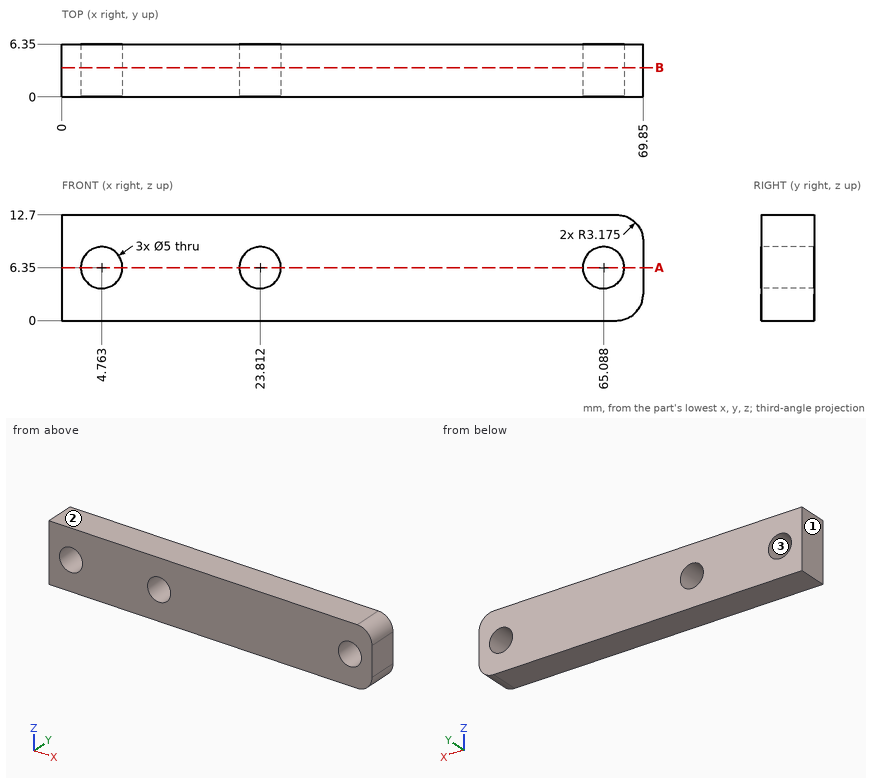
Here's the drawing with two shaded views (mm, measured from the low corner). I have some questions. Coordinates: 2 decimals unless noted, no trailing zeros. Loops run counter-clockwise (first coordinate to the right, second up) from the corner with the lowest first, then second, coordinate; pieces in that order, holes last. Notation, with made-up numbers: (-7.75, -13.5) -> (1.25, -13.5) arc R20 ccw to (1.25, 6.5) -> close; hole circle Ø10 at (-26.5, -14). An arc over 180 degrees is marked (long way). Answer as a JSON object with one key per item and string values.
1) Thinking about a two-plate mould opening in Z: for the marked faces 1, 2 and 3, which applies, pulls with the +Z half, pulls with the -Z half, needs draft (parallel to the pull), parting line crosses it, or undercut?
Results:
{"face 1": "needs draft", "face 2": "pulls with the +Z half", "face 3": "undercut"}
2) If I drill on line 1 (Z direction, x = 24, y = 2.25); line 2 (X direction, y = 2.25, z = 3) (1 decimal); line 3 (X direction, y = 5.5, z = 10.75) (1 decimal), over which ranges is the centre line in solid material (lowest first)?
Results:
{"line 1": "z = 0 to 3.86, 8.84 to 12.7", "line 2": "x = 0 to 69.8", "line 3": "x = 0 to 69.6"}
3) Imagine slicing it at B-B (y = 3.5). Count the separate pieces of the cut face and the enclosed holes in it, then the cut area to 3 significant figures.
Results:
{"separate pieces": "1", "enclosed holes": "3", "area": "824 mm^2"}
4) Imagine slicing it at A-A (z = 6.35). Please give me the cut outline in (x, y), then the cut area to 3 significant figures.
Results:
{"outline": "(0, 0) -> (2.26, 0) -> (2.26, 6.35) -> (0, 6.35) -> close; (7.26, 0) -> (21.31, 0) -> (21.31, 6.35) -> (7.26, 6.35) -> close; (26.31, 0) -> (62.59, 0) -> (62.59, 6.35) -> (26.31, 6.35) -> close; (67.59, 0) -> (69.85, 0) -> (69.85, 6.35) -> (67.59, 6.35) -> close", "area": "348 mm^2"}
5) For P1, Ø3, axis at x = 23.81, z = 6.35, coming from the -Y side, with a flat end and sliding along its axis, tell me the tip position at first contact or that it passes through.
Results:
{"P1": "passes through"}
